Read the model definition and answer for the solid it produces. Units are mm, in the model's axes. Face numbers are marked on the shaded views. A direction names the side the tool comes from. Coordinates: 2 decimals unless noted, no trailing zeros. Loops run counter-clockwise (first coordinate to the right, second up) from the corner with the lowest first, then second, coordinate; pieces in that order, holes last. Notation, with made-up numbers: (10, -5.5) -> (63, -5.5) arc R10 cw to (63, 0.5) -> close; hole circle Ø2 at (55, 86). An arc over 180 degrees is marked (long way). Answer as a JSON object with one key per item and string values. Group by question number.
Q1. Straight lines are drawn through the part: line 1 along X through (y, z) = (-7, 58.5); line 2 along X through (y, z) = (-46.5, 114); line 3 along Z through (x, y) = (-21, -5.5). For each, find the intervals that lie inside material, in ascending order. Write a range as [from, to].
Q2. Each of these flat-tipped pins is pushed along its axis until it touches: P1, Ø4.5, axis at y = -65, z = 35, coming from the -X side; P2, Ø7, axis at y = -19, z = 85, coming from the -X side; P3, Ø6, axis at x = -29, z = 47, coming from the -Y side. Where does it stop, or does it pass through?
Q3. The part is cut by section A-A on z = 60. Write down the section's boundary in (x, y).
Q4. The part is cut by section C-C on z = 7. Write down the section's boundary in (x, y), and give its area (3 significant figures).
Q5. The part is cut by section B-B on x = -42. Write down the section's boundary in (y, z).
Q6. The part is cut by section D-D on y = -19. Write down the section's boundary in (x, z), and give its area (3 significant figures).
Q7. For the marked faces 1 and 2, determine the directions among +Z, -Z, +X, -X, +Y, -Y from which every point of the face is accessible in a straight line to the end or side of a thin tool.
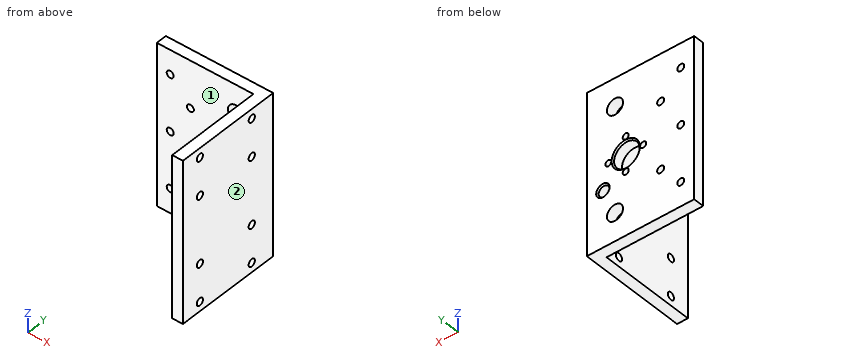
from build123d import *

# Parameters (mm, degrees)
ESTRUSIONE_ESTRUSIONE1_DEPTH = 120
TAGLIO_ESTRUSIONE2_REACH     = 166.924
SCHIZZO6_R                   = 6
TAGLIO_ESTRUSIONE3_REACH     = 166.924
SCHIZZO7_R                   = 9.5
SCHIZZO7_R_2                 = 4
FORO_PER_VITE_M4_2_D         = 4.5
SCHIZZO12_R                  = 2.75
TAGLIO_ESTRUSIONE4_DEPTH     = 10
SCHIZZO14_R                  = 2.6
TAGLIO_ESTRUSIONE5_DEPTH     = 10
SMUSSO1_SIZE                 = 1
SMUSSO2_SIZE                 = 1


with BuildPart() as part:
    # Schizzo1 → Estrusione-Estrusione1 (new body)
    with BuildSketch(Plane.XY):
        Polygon((0, 0), (-80, 0), (-80, -8), (-8, -8), (-8, -80), (0, -80), align=None)
    extrude(amount=ESTRUSIONE_ESTRUSIONE1_DEPTH)

    # Schizzo6 → Taglio-Estrusione2 (cut, up to next)
    with BuildSketch(Plane(origin=(0, 0, 0), x_dir=(1, 0, 0), z_dir=(0, 1, 0)), mode=Mode.PRIVATE) as taglio_estrusione2_sk1:
        with Locations(Location((-21, -21, 0), (0, 0, 180))):
            Circle(SCHIZZO6_R)
    taglio_estrusione2_tool1 = extrude(taglio_estrusione2_sk1.sketch, amount=-TAGLIO_ESTRUSIONE2_REACH, mode=Mode.PRIVATE) & part.part
    # Schizzo6 → Taglio-Estrusione2 (cut, up to next)
    with BuildSketch(Plane(origin=(0, 0, 0), x_dir=(1, 0, 0), z_dir=(0, 1, 0)), mode=Mode.PRIVATE) as taglio_estrusione2_sk2:
        with Locations(Location((-21, -99, 0), (0, 0, 180))):
            Circle(SCHIZZO6_R)
    taglio_estrusione2_tool2 = extrude(taglio_estrusione2_sk2.sketch, amount=-TAGLIO_ESTRUSIONE2_REACH, mode=Mode.PRIVATE) & part.part
    add(taglio_estrusione2_tool1.solids().sort_by_distance((-21, 0, 21))[0], mode=Mode.SUBTRACT)
    add(taglio_estrusione2_tool2.solids().sort_by_distance((-21, 0, 99))[0], mode=Mode.SUBTRACT)

    # Schizzo7 → Taglio-Estrusione3 (cut, up to next)
    with BuildSketch(Plane(origin=(0, 0, 0), x_dir=(1, 0, 0), z_dir=(0, 1, 0)), mode=Mode.PRIVATE) as taglio_estrusione3_sk1:
        with Locations(Location((-29, -60, 0), (0, 0, 180))):
            Circle(SCHIZZO7_R)
    taglio_estrusione3_tool1 = extrude(taglio_estrusione3_sk1.sketch, amount=-TAGLIO_ESTRUSIONE3_REACH, mode=Mode.PRIVATE) & part.part
    # Schizzo7 → Taglio-Estrusione3 (cut, up to next)
    with BuildSketch(Plane(origin=(0, 0, 0), x_dir=(1, 0, 0), z_dir=(0, 1, 0)), mode=Mode.PRIVATE) as taglio_estrusione3_sk2:
        with Locations(Location((-12, -42, 0), (0, 0, 180))):
            Circle(SCHIZZO7_R_2)
    taglio_estrusione3_tool2 = extrude(taglio_estrusione3_sk2.sketch, amount=-TAGLIO_ESTRUSIONE3_REACH, mode=Mode.PRIVATE) & part.part
    add(taglio_estrusione3_tool1.solids().sort_by_distance((-29, 0, 60))[0], mode=Mode.SUBTRACT)
    add(taglio_estrusione3_tool2.solids().sort_by_distance((-12, 0, 42))[0], mode=Mode.SUBTRACT)

    # Foro per Vite M4-2 (through all)
    with Locations(Plane(origin=(0, 0, 0), x_dir=(1, 0, 0), z_dir=(0, 1, 0))):
        with Locations((-29, -47), (-42, -60), (-29, -73), (-16, -60), (-29, -60)):
            Hole(FORO_PER_VITE_M4_2_D / 2)

    # Schizzo12 → Taglio-Estrusione4 (cut)
    with BuildSketch(Plane(origin=(0, 0, 0), x_dir=(0, 0, -1), z_dir=(1, 0, 0))):
        with Locations((-113, -19)):
            Circle(SCHIZZO12_R)
        with Locations(Location((-85, -19, 0), (0, 0, 90))):
            Circle(SCHIZZO12_R)
        with Locations((-35, -19)):
            Circle(SCHIZZO12_R)
        with Locations(Location((-7, -19, 0), (0, 0, 90))):
            Circle(SCHIZZO12_R)
        with Locations((-85, -65)):
            Circle(SCHIZZO12_R)
        with Locations(Location((-113, -65, 0), (0, 0, 90))):
            Circle(SCHIZZO12_R)
        with Locations((-7, -65)):
            Circle(SCHIZZO12_R)
        with Locations(Location((-35, -65, 0), (0, 0, 90))):
            Circle(SCHIZZO12_R)
    extrude(amount=-TAGLIO_ESTRUSIONE4_DEPTH, mode=Mode.SUBTRACT)

    # Schizzo14 → Taglio-Estrusione5 (cut)
    with BuildSketch(Plane(origin=(0, 0, 0), x_dir=(1, 0, 0), z_dir=(0, 1, 0))):
        with Locations(Location((-70, -18, 0), (0, 0, 180))):
            Circle(SCHIZZO14_R)
        with Locations(Location((-70, -60, 0), (0, 0, 180))):
            Circle(SCHIZZO14_R)
        with Locations(Location((-70, -102, 0), (0, 0, 180))):
            Circle(SCHIZZO14_R)
        with Locations(Location((-55, -35, 0), (0, 0, 180))):
            Circle(SCHIZZO14_R)
        with Locations(Location((-55, -85, 0), (0, 0, 180))):
            Circle(SCHIZZO14_R)
    extrude(amount=-TAGLIO_ESTRUSIONE5_DEPTH, mode=Mode.SUBTRACT)

    # Smusso1
    smusso1_edges = [part.edges().sort_by_distance(p)[0] for p in [
        (-8, 0, 42),
    ]]
    chamfer(smusso1_edges, length=SMUSSO1_SIZE)

    # Smusso2
    smusso2_edges = [part.edges().sort_by_distance(p)[0] for p in [
        (-19.5, 0, 60),
    ]]
    chamfer(smusso2_edges, length=SMUSSO2_SIZE)


solid = part.part
Final values:
{
 "1": {"line 1": "x = [-80, -72.12], [-67.88, -43.68], [-40.32, -38.38], [-19.62, -17.68], [-14.32, 0]", "line 2": "x = [-8, 0]", "line 3": "z = [0, 15], [27, 54.88], [65.12, 93], [105, 120]"},
 "2": {"P1": "passes through", "P2": "stops at x = -8", "P3": "stops at y = -8"},
 "3": {"outline": "(-80, -8) -> (-72.6, -8) -> (-72.6, 0) -> (-80, 0) -> close; (-67.4, -8) -> (-44.25, -8) -> (-44.25, 0) -> (-67.4, 0) -> close; (-39.75, -8) -> (-38.5, -8) -> (-38.5, -1) -> (-39.5, 0) -> (-39.75, 0) -> close; (-19.5, -8) -> (-18.25, -8) -> (-18.25, 0) -> (-18.5, 0) -> (-19.5, -1) -> close; (-13.75, -8) -> (-8, -8) -> (-8, -80) -> (0, -80) -> (0, 0) -> (-13.75, 0) -> close"},
 "4": {"outline": "(-80, -8) -> (-8, -8) -> (-8, -16.25) -> (0, -16.25) -> (0, 0) -> (-80, 0) -> close; (-8, -80) -> (0, -80) -> (0, -67.75) -> (-8, -67.75) -> close; (-8, -62.25) -> (0, -62.25) -> (0, -21.75) -> (-8, -21.75) -> close", "area": "1,130 mm2"},
 "5": {"outline": "(-8, 0) -> (0, 0) -> (0, 57.75) -> (-8, 57.75) -> close; (-8, 62.25) -> (0, 62.25) -> (0, 120) -> (-8, 120) -> close"},
 "6": {"outline": "(-8, 0) -> (0, 0) -> (0, 4.25) -> (-8, 4.25) -> close; (-8, 9.75) -> (0, 9.75) -> (0, 32.25) -> (-8, 32.25) -> close; (-8, 37.75) -> (0, 37.75) -> (0, 82.25) -> (-8, 82.25) -> close; (-8, 87.75) -> (0, 87.75) -> (0, 110.25) -> (-8, 110.25) -> close; (-8, 115.75) -> (0, 115.75) -> (0, 120) -> (-8, 120) -> close", "area": "784 mm2"},
 "7": {"face 1": "+Z, -Z, -X, -Y", "face 2": "+Z, -Z, +X, +Y, -Y"}
}
